from build123d import *

# Parameters (mm, degrees)
SKETCH1_R           = 1.8288
SKETCH1_R_2         = 4.7625
BOSS_EXTRUDE1_DEPTH = 3.175
CUT_EXTRUDE1_DEPTH  = 107.506615522
FILLET1_R           = 2.5
FILLET2_R           = 5


with BuildPart() as part:
    # Sketch1 → Boss-Extrude1 (new body)
    with BuildSketch(Plane(origin=(0, 0, 0), x_dir=(0, 0, -1), z_dir=(1, 0, 0))):
        with BuildLine():
            Line((-16.645, -105.15), (16.645, -105.15))
            Line((16.645, -105.15), (16.645, 5.15))
            Line((16.645, 5.15), (6.94973031, 37.108353593))
            ThreePointArc((6.94973031, 37.108353593), (0, 42.2625), (-6.94973031, 37.108353593))
            Line((-6.94973031, 37.108353593), (-16.645, 5.15))
            Line((-16.645, 5.15), (-16.645, -105.15))
        make_face()
        with Locations((-13.4747, 0)):
            Circle(SKETCH1_R, mode=Mode.SUBTRACT)
        with Locations((0, 35)):
            Circle(SKETCH1_R_2, mode=Mode.SUBTRACT)
        with Locations((13.4747, 0)):
            Circle(SKETCH1_R, mode=Mode.SUBTRACT)
        with Locations((-13.4747, -100)):
            Circle(SKETCH1_R, mode=Mode.SUBTRACT)
        with Locations((13.4747, -100)):
            Circle(SKETCH1_R, mode=Mode.SUBTRACT)
    extrude(amount=BOSS_EXTRUDE1_DEPTH)

    # Sketch2 → Cut-Extrude1 (cut, through all)
    with BuildSketch(Plane(origin=(3.175, 0, 0), x_dir=(0, 0, -1), z_dir=(1, 0, 0))):
        Polygon((11.645, -2.5), (-11.645, -2.5), (11.645, -26.898674048), align=None)
        Polygon((-11.645, -9.741325952), (11.645, -34.14), (-11.645, -58.538674048), (-11.645, -34.14), align=None)
        Polygon((-11.645, -73.021325952), (-11.645, -97.42), (11.645, -97.42), align=None)
        Polygon((11.645, -41.381325952), (11.645, -65.78), (11.645, -90.178674048), (-11.645, -65.78), align=None)
    extrude(amount=-CUT_EXTRUDE1_DEPTH, mode=Mode.SUBTRACT)

    # Fillet1
    fillet1_edges = [part.edges().sort_by_distance(p)[0] for p in [
        (1.5875, -9.741325952, 11.645),
        (1.5875, -34.14, -11.645),
        (1.5875, -58.538674048, 11.645),
        (1.5875, -26.898674048, -11.645),
        (1.5875, -2.5, 11.645),
        (1.5875, -2.5, -11.645),
        (1.5875, -90.178674048, -11.645),
        (1.5875, -65.78, 11.645),
        (1.5875, -41.381325952, -11.645),
        (1.5875, -73.021325952, 11.645),
        (1.5875, -97.42, -11.645),
        (1.5875, -97.42, 11.645),
    ]]
    fillet(fillet1_edges, radius=FILLET1_R)

    # Fillet2
    fillet2_edges = [part.edges().sort_by_distance(p)[0] for p in [
        (1.5875, -105.15, -16.645),
        (1.5875, -105.15, 16.645),
        (1.5875, 5.15, 16.645),
        (1.5875, 5.15, -16.645),
    ]]
    fillet(fillet2_edges, radius=FILLET2_R)


solid = part.part
Geometry check sheet. Reference: the model listing, model coordinates, mm. A direction names the side the tool comes from. Round coordinates to 2 decimals unless told otherwise and drop trailing zeros. Order: outer loops, then holes, each group sorted by start corner. A loop starts at its lowest first (then second) coordinate and runs counter-clockwise, first axis right, second up. Notation, with made-up numbers: M 27,-11.5 L 60,-11.5 A29 ccw 60,16.5 Z; hole C 70.25,64 d1. An arc over 180 degrees is marked long. Answer in a Markdown table with one row per item. Add a question column.
Item 1: Sectioned sample at A-A, the plane y = 0. Enter the section's corners in (x, z) (1 decimal), plus the area to 3 significant figures.
Item 2: Set-up check for faces 1 (the face through (0, -14, 4)), 2 (the face through (1.565, -13.676, 10.113)): record each of +Z, -Z, +X, -X, +Y, -Y from which the full face is reachable in a straight line by a thin tool's end or side.
Item 3: Sectioned sample at B-B, the plane z = 0. State how many separate pieces and enclosed holes the cut face has, plus the area to 3 significant figures.
Item 4: Sectioned sample at C-C, the plane y = 35. Enter the section's corners in (x, z) (1 decimal), plus the area to 3 significant figures.
Item 5: Material ranges on L1, parallel to Z at x = 1.2, y = -100 (1 decimal); L2, parallel to Y at x = 1.9, z = 2; L3, parallel to Z at x = 0.8, y = -22 (3 decimals), recorded low to high. Write a range as [from, to].
Item 6: Depth check by flat-ended pin: pin 1 Ø1.6 at (x, z) = (1.5, 4) entering from +Y; pin 2 Ø1 at (x, z) = (2, -2) entering from +Y. Enter the tip coordinate at first touch or a pass-through.
Item 7: Draft check along Z on faces 3 (the face through (1.61, -103.724, 15.141)), 4 (the face through (2, -49, -16.645)), 5 (the face through (3.175, -14, 4)), 6 (the face through (1.57, -101.62, 12.63)). Enter one of: released by +Z, released by -Z, zero draft, split by the parting line, or undercut.
Filled in:
| question | item | result |
|---|---|---|
| 1 | outline | M 0,-16.6 L 3.2,-16.6 L 3.2,-15.3 L 0,-15.3 Z; M 0,-11.6 L 3.2,-11.6 L 3.2,11.6 L 0,11.6 Z; M 0,15.3 L 3.2,15.3 L 3.2,16.6 L 0,16.6 Z |
| 1 | area | 82.5 mm² |
| 2 | face 1 | +Z, -Z, -X, +Y, -Y |
| 2 | face 2 | +X, -X |
| 3 | separate pieces | 6 |
| 3 | enclosed holes | 0 |
| 3 | area | 205 mm² |
| 4 | outline | M 0,-7.6 L 3.2,-7.6 L 3.2,-4.8 L 0,-4.8 Z; M 0,4.8 L 3.2,4.8 L 3.2,7.6 L 0,7.6 Z |
| 4 | area | 18.0 mm² |
| 5 | L1 | z = [-16.6, -15.3], [-11.6, 11.6], [15.3, 16.6] |
| 5 | L2 | y = [-105.15, -97.42], [-83.13, -75.88], [-55.68, -48.43], [-19.85, -12.6], [-2.5, 30.68], [39.32, 41.98] |
| 5 | L3 | z = [-16.645, -11.255], [-6.969, -0.057], [11.645, 16.645] |
| 6 | pin 1 | stops at y = 41.52 |
| 6 | pin 2 | stops at y = 42.11 |
| 7 | face 3 | released by +Z |
| 7 | face 4 | released by -Z |
| 7 | face 5 | zero draft |
| 7 | face 6 | undercut |
